Source: CAD feature listing. Evaluate the final solid. Frame: model axes, mm. Round coordinates to 2 decimals unless told otherwise and drop trailing zeros. Loops run counter-clockwise (first coordinate to the right, second up) from the corner with the lowest first, then second, coordinate; pieces in that order, holes last. Notation, with made-up numbers: (46, 44.25) - (97, 44.25) arc R24 cw to (97, 65.25) - close; hole circle Ø2 at (69.25, -40). An arc over 180 degrees is marked (long way). One line per question, with ' | ' between items.
Autodesk Inventor part; units mm, degrees
ref_plane "YZ Plane" through (0, 0, 0) normal (1, 0, 0) x (0, 1, 0)
ref_plane "XZ Plane" through (0, 0, 0) normal (0, 1, 0) x (-1, 0, 0)
ref_plane "XY Plane" through (0, 0, 0) normal (0, 0, 1) x (1, 0, 0)
sketch "Sketch1" plane through (0, 0, 0) normal (0, 1, 0) x (-1, 0, 0)
  circle A0 centre (0, 0) radius 73.025
  line L0 (0, 0) -> (0, -73.025) construction
  line L1 (0, 0) -> (-12.6807, -71.9156)
  line L2 (0, 0) -> (12.6807, -71.9156)
  line L3 (0, 0) -> (72.3143, -10.1631)
  line L4 (0, 0) -> (64.4772, -34.2832)
  line L5 (0, 0) -> (32.0121, 65.6344)
  line L6 (0, 0) -> (52.5298, 50.7274)
  line L7 (0, 0) -> (-52.5298, 50.7274)
  line L8 (0, 0) -> (-32.0121, 65.6344)
  line L9 (0, 0) -> (-64.4772, -34.2832)
  line L10 (0, 0) -> (-72.3143, -10.1631)
  circle A1 centre (0, 0) radius 69.85
  arc A2 (4.7597, -69.6876) -> (-4.7597, -69.6876) centre (0, -69.85) ccw
  arc A3 (67.7477, -17.0079) -> (64.806, -26.0614) centre (66.4313, -21.5848) ccw
  arc A4 (37.1107, 59.1762) -> (44.8121, 53.5808) centre (41.0568, 56.5098) ccw
  arc A5 (-44.8121, 53.5808) -> (-37.1107, 59.1762) centre (-41.0568, 56.5098) ccw
  arc A6 (-64.806, -26.0614) -> (-67.7477, -17.0079) centre (-66.4313, -21.5848) ccw
  point P0 (61.6739, -32.7926)
  point P1 (69.1702, -9.7212)
  point P2 (50.2459, 48.5219)
  point P3 (30.6202, 62.7808)
  point P4 (-30.6202, 62.7808)
  point P5 (-50.2459, 48.5219)
  point P6 (-69.1702, -9.7212)
  point P7 (-61.6739, -32.7926)
  point P8 (-12.1293, -68.7888)
  point P9 (12.1293, -68.7888)
  point P10 (64.806, -26.0614)
  point P11 (67.7477, -17.0079)
  point P12 (44.8121, 53.5808)
  point P13 (37.1107, 59.1762)
  point P14 (-37.1107, 59.1762)
  point P15 (-67.7477, -17.0079)
  dimension "d0" = 146.05
  dimension "d1" = 10
  dimension "d4" = 360
  dimension "d6" = 3.175
  dimension "d10" = 9.525
  dimension "d13" = 360
extrude "Extrusion1" add sketch "Sketch1" along normal blind 1.5875 contours A0 L3 A1 L6 | L5 A1 L8 A0 | A1 L3 L6 | L6 L5 A1 A4 | A0 L2 A1 L4 | A1 A3 L4 L3 | L5 L8 A1 | L2 A1 A2 L1 | L4 A1 L2 | L10 A1 L7 | L7 A1 A5 L8 | L1 A1 L9 | L9 A1 A6 L10 | L7 A1 L10 A0 | L1 A0 L9 A1
fillet "Fillet1" radius 1.5875 30 edges at (30.6202, 0.7937, 62.7808) (32.0121, 0.7937, 65.6344) (-30.6202, 0.7937, 62.7808) (-32.0121, 0.7937, 65.6344) (-52.5298, 0.7937, 50.7274) (-50.2459, 0.7937, 48.5219) (52.5298, 0.7937, 50.7274) (50.2459, 0.7937, 48.5219) (64.4772, 0.7937, -34.2832) (61.6739, 0.7937, -32.7926) (72.3143, 0.7937, -10.1631) (69.1702, 0.7937, -9.7212) (12.6807, 0.7937, -71.9156) (12.1293, 0.7937, -68.7888) (-12.6807, 0.7937, -71.9156) (-12.1293, 0.7937, -68.7888) (-72.3143, 0.7937, -10.1631) (-69.1702, 0.7937, -9.7212) (-64.4772, 0.7937, -34.2832) (-61.6739, 0.7937, -32.7926) (37.1107, 0.7937, 59.1762) (44.8121, 0.7937, 53.5808) (-44.8121, 0.7937, 53.5808) (-37.1107, 0.7937, 59.1762) (-64.806, 0.7937, -26.0614) (-67.7477, 0.7937, -17.0079) (4.7597, 0.7937, -69.6876) (-4.7597, 0.7937, -69.6876) (67.7477, 0.7937, -17.0079) (64.806, 0.7937, -26.0614)
sketch "Sketch5" plane through (0, 1.5875, 0) normal (0, 1, 0) x (1, 0, 0)
  line L0 (0, 0) -> (0, 65.0875) construction
  arc A0 (-4.554, 68.4564) -> (4.554, 68.4564) centre (0, 69.85) ccw
  circle A1 centre (0, 50.8) radius 22.225
  arc A2 (63.6995, 35.7075) -> (14.2757, 71.616) centre (0, 0) ccw
  circle A3 centre (0, 50.8) radius 12.5 construction
  circle A4 centre (-24.6062, 60.325) radius 1.7526
  circle A5 centre (-24.6062, 60.325) radius 3.175 construction
  circle A6 centre (-22.225, 34.925) radius 3.175
  circle A7 centre (-22.225, 34.925) radius 1.7526
  circle A8 centre (24.6062, 60.325) radius 1.7526
  circle A9 centre (24.6062, 60.325) radius 3.175
  circle A10 centre (22.225, 34.925) radius 3.175
  circle A11 centre (22.225, 34.925) radius 1.7526
  arc A12 (6.2133, 69.5731) -> (4.554, 68.4564) centre (6.0721, 67.9919) ccw
  arc A13 (6.2133, 69.5731) -> (4.554, 68.4564) centre (6.0721, 67.9919) ccw
  arc A14 (-4.554, 68.4564) -> (-6.2133, 69.5731) centre (-6.0721, 67.9919) ccw
  arc A15 (-4.554, 68.4564) -> (-6.2133, 69.5731) centre (-6.0721, 67.9919) ccw
  arc A16 (-12.4019, 70.3348) -> (-10.5977, 69.0414) centre (-10.8385, 70.6105) ccw
  arc A17 (10.5977, 69.0414) -> (12.4019, 70.3348) centre (10.8385, 70.6105) ccw
  arc A18 (10.5977, 69.0414) -> (6.2133, 69.5731) centre (0, 0) ccw
  arc A19 (10.5977, 69.0414) -> (11.9875, 69.515) centre (10.8385, 70.6105) ccw
  arc A20 (-6.2133, 69.5731) -> (-10.5977, 69.0414) centre (0, 0) ccw
  arc A21 (-14.2757, 71.616) -> (-63.6995, 35.7075) centre (0, 0) ccw
  line L1 (-28.4451, 67.2572) -> (-25.3861, 34.6286)
  line L2 (-22.7046, 31.7864) -> (-3.3572, 28.83)
  line L3 (28.4451, 67.2572) -> (25.3861, 34.6286)
  line L4 (22.7046, 31.7864) -> (3.3572, 28.83)
  circle A22 centre (0, 63.3) radius 1.5
  circle A23 centre (-12.5, 50.8) radius 1.5
  circle A24 centre (0, 38.3) radius 1.5
  circle A25 centre (12.5, 50.8) radius 1.5
  circle A26 centre (0, 50.8) radius 6.35
  circle A27 centre (0, 0) radius 73.025
  point P0 (-63.6995, 35.7075)
  dimension "d39" = 25
  dimension "d40" = 44.45
  dimension "d41" = 3.5052
  dimension "d42" = 6.35
  dimension "d43" = 9.525
  dimension "d44" = 24.6062
  dimension "d45" = 6.35
  dimension "d46" = 3.5052
  dimension "d47" = 15.875
  dimension "d48" = 22.225
  dimension "d63" = 3
  dimension "d66" = 360
  dimension "d68" = 12.7
extrude "Extrusion3" cut sketch "Sketch5" against normal blind 25.4 contours A1 L4 A10 L3 A2 A27 A21 L1 A6 L2 | A4 | A7 | A8 | A11 | A22 | A23 | A24 | A25 | A26
fillet "Fillet4" radius 6.35 2 edges at (-28.4451, 0.7937, -67.2572) (28.4451, 0.7937, -67.2572)
equation "\"d45\" = d42"
equation "\"d46\" = d41"
properties part number "Top Plate" material "Aluminum 6061"
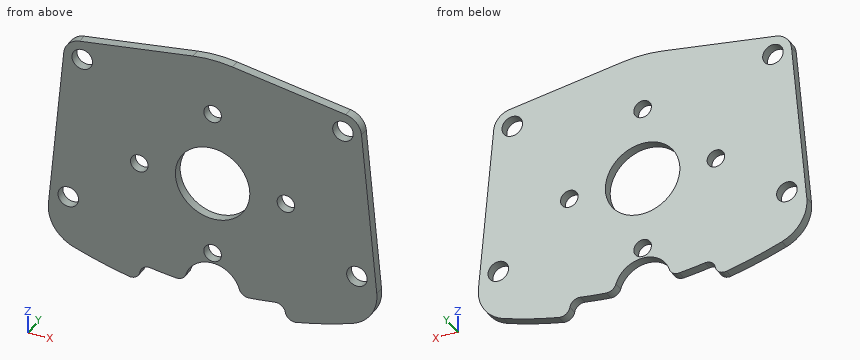
1. Material intervals for probe 1 along Z at (x, y) = (0, 0.7) (3 decimals); probe 2 along X at (y, z) = (0.5, -63.3); probe 3 along X at (y, z) = (0.25, -35.5), sorted ascending.
Worked out:
probe 1: z = -65.088 to -64.8, -61.8 to -57.15, -44.45 to -39.8, -36.8 to -28.575 | probe 2: x = -28.02 to -1.5, 1.5 to 28.02 | probe 3: x = -25.47 to -23.88, -20.57 to 20.57, 23.88 to 25.47
2. Section query B-B, the plane z = -45.5. Return loops of the section in (x, y).
Worked out:
outline: (-26.41, 0) - (-3.5, 0) - (-3.5, 1.59) - (-26.41, 1.59) - close; (3.5, 0) - (26.41, 0) - (26.41, 1.59) - (3.5, 1.59) - close
3. Section query C-C, the plane z = -50.8. Return loops of the section in (x, y), plus the area to 3 significant figures.
Worked out:
outline: (-26.9, 0) - (-14, 0) - (-14, 1.59) - (-26.9, 1.59) - close; (-11, 0) - (-6.35, 0) - (-6.35, 1.59) - (-11, 1.59) - close; (6.35, 0) - (11, 0) - (11, 1.59) - (6.35, 1.59) - close; (14, 0) - (26.9, 0) - (26.9, 1.59) - (14, 1.59) - close | area: 55.7 mm2
4. Contact query for a flat-ended pin moving along its axis: P1, Ø3.5, axis at x = 0, z = -63.3, coming from the -Y side. Output: stop coordinate, or through.
Worked out:
P1: stops at y = 0
5. Section query A-A, the plane x = 2.5. Return loops of the section in (y, z), plus the area to 3 significant figures.
Worked out:
outline: (0, -65.8) - (1.59, -65.8) - (1.59, -56.64) - (0, -56.64) - close; (0, -44.96) - (1.59, -44.96) - (1.59, -28.72) - (0, -28.72) - close | area: 40.3 mm2
6. Section query D-D, the plane y = 0.7. Give the number of separate pieces and of enclosed holes in the cut face, plus the area to 3 significant figures.
Worked out:
separate pieces: 1 | enclosed holes: 9 | area: 1,880 mm2
